Source: CAD feature listing. Evaluate the final solid. Frame: model axes, mm. A direction names the side the tool comes from. Round coordinates to 2 decimals unless told otherwise and drop trailing zeros. Loops run counter-clockwise (first coordinate to the right, second up) from the corner with the lowest first, then second, coordinate; pieces in that order, holes last.
Item 1: Section query C-C on y = -0.5. Return loops of the section in (x, z).
Item 2: Section query A-A on x = -23. Return loops of the section in (y, z), then the cut area to 3 significant figures.
Item 3: Section query D-D on z = 11. Give the number of separate pieces and of enclosed holes in the cut face, then the cut area to 3 significant figures.
Item 4: Pull-direction query (X, two-part tool) for faces 5 (the flat face through (14, 20, 13)), 6 (the cylindrical face through (7.18, 4.75, 11.9)), 7 (the flat face through (-26.86, 10.315, 48.479)); classes: released by +X, released by -X, zero draft, split by the parting line, or undercut.
Item 5: Access query for faces 1 (the flat face through (36, 28, 13)), 2 (the flat face through (31, -2.471, 48)), 3 (the flat face through (15, 18, 10)), 4 (the flat face through (36.1, 24.6, 50)). Directions: +Z, -Z, +X, -X, +Y, -Y. A direction counts if a zero-diameter tool reaches every point of the face in a straight line with its end or side. Return the directions, or none.
Item 6: Section query B-B on z = 39. Return loops of the section in (x, y).
Item 7: First-contact query: P1, Ø5, axis at x = 31, z = 10, coming from the +Y side; P2, Ø1.9, axis at x = 4.32, z = 11, coming from the -Y side; P3, Ø8, axis at x = 16.5, y = 21.5, coming from the -Z side; P4, Ø1, axis at x = 20.5, z = 14, coming from the +Y side. Flat tips, straight axial feed; report the tip coordinate or a pass-through.
Item 8: Ray query, L1, parallel to Z at x = 34, y = 26.5; L2, parallel to X at y = 1.5, z = 47.5 (3 decimals); L3, parallel to Z at x = 5, y = 11. Return the intervals inside material, ascending.
```python
from build123d import *

# Parameters (mm, degrees)
EXTRUDE_1_DEPTH     = 60
SKETCH_2_W          = 32.5
SKETCH_2_H          = 3
EXTRUDE_2_DEPTH     = 8.5
SKETCH_3_W          = 32.5
SKETCH_3_H          = 34
EXTRUDE_3_DEPTH     = 1
SKETCH_4_R          = 2.4
CUT_EXTRUDE_1_DEPTH = 100
CUT_EXTRUDE_3_DEPTH = 100
SKETCH_5_R          = 1.62
CUT_EXTRUDE_4_DEPTH = 100
SKETCH_7_R          = 3
CUT_EXTRUDE_5_DEPTH = 100


with BuildPart() as part:
    # 草图1 → 凸台-拉伸1 (new body)
    with BuildSketch(Plane.XY):
        Polygon((-38.683076923, -5.470769231), (45.316923077, -5.470769231), (45.244014743, 20.991341126), (44.341897344, 23.852491978), (-39.585194322, -2.609618379), align=None)
    extrude(amount=EXTRUDE_1_DEPTH)

    # 草图2 → 凸台-拉伸2 (add)
    with BuildSketch(Plane(origin=(-2.83104293, 8.978921042, 0), x_dir=(0.9537169507482267, 0.30070579950427384, 0), z_dir=(-0.30070579950427384, 0.9537169507482267, 0))):
        with Locations((-22.287798204, -11.5)):
            Rectangle(SKETCH_2_W, SKETCH_2_H)
        with Locations((-22.287798204, -48.5)):
            Rectangle(SKETCH_2_W, SKETCH_2_H)
        with Locations((33.212201796, -11.5)):
            Rectangle(SKETCH_2_W, SKETCH_2_H)
        with Locations((33.212201796, -48.5)):
            Rectangle(SKETCH_2_W, SKETCH_2_H)
    extrude(amount=EXTRUDE_2_DEPTH)

    # 草图3 → 凸台-拉伸3 (add)
    with BuildSketch(Plane(origin=(-2.83104293, 8.978921042, 0), x_dir=(0.9537169507482267, 0.30070579950427384, 0), z_dir=(-0.30070579950427384, 0.9537169507482267, 0))):
        with Locations((-22.287798204, -30)):
            Rectangle(SKETCH_3_W, SKETCH_3_H)
        with Locations((33.212201796, -30)):
            Rectangle(SKETCH_3_W, SKETCH_3_H)
    extrude(amount=EXTRUDE_3_DEPTH)

    # 草图4 → 切除-拉伸1 (cut)
    with BuildSketch(Plane.XY.offset(50)):
        with Locations((-35.850165862, 3.003309771)):
            Circle(SKETCH_4_R)
        with Locations((-14.874407062, 9.637911699)):
            Circle(SKETCH_4_R)
        with Locations((17.075110788, 19.711555982)):
            Circle(SKETCH_4_R)
        with Locations((38.056883705, 26.327083571)):
            Circle(SKETCH_4_R)
    extrude(amount=-CUT_EXTRUDE_1_DEPTH, mode=Mode.SUBTRACT)

    # 草图6 → 切除-拉伸3 (cut)
    with BuildSketch(Plane(origin=(0, 0, 10), x_dir=(-1, 0, 0), z_dir=(0, 0, -1))):
        Polygon((-31.771870066, 28.801675164), (-34.327869361, 20.695081083), (-23.360124428, 17.236964389), (-20.804125132, 25.34355847), align=None)
    extrude(amount=-CUT_EXTRUDE_3_DEPTH, mode=Mode.SUBTRACT)

    # 草图5 → 切除-拉伸4 (cut)
    with BuildSketch(Plane(origin=(0, -5.470769231, 0), x_dir=(-1, 0, 0), z_dir=(0, -1, 0))):
        with Locations(Location((-29.316923077, -49, 0), (0, 0, 180))):
            Circle(SKETCH_5_R)
        with Locations(Location((-29.316923077, -11, 0), (0, 0, 180))):
            Circle(SKETCH_5_R)
        with Locations(Location((-4.316923077, -49, 0), (0, 0, 180))):
            Circle(SKETCH_5_R)
        with Locations(Location((-4.316923077, -11, 0), (0, 0, 180))):
            Circle(SKETCH_5_R)
    extrude(amount=-CUT_EXTRUDE_4_DEPTH, mode=Mode.SUBTRACT)

    # 草图7 → 切除-拉伸5 (cut)
    with BuildSketch(Plane(origin=(0, -2.470769231, 0), x_dir=(-1, 0, 0), z_dir=(0, -1, 0))):
        with Locations(Location((-29.316923077, -11, 0), (0, 0, 180))):
            Circle(SKETCH_7_R)
        with Locations(Location((-4.316923077, -11, 0), (0, 0, 180))):
            Circle(SKETCH_7_R)
        with Locations(Location((-29.316923077, -49, 0), (0, 0, 180))):
            Circle(SKETCH_7_R)
        with Locations(Location((-4.316923077, -49, 0), (0, 0, 180))):
            Circle(SKETCH_7_R)
    extrude(amount=-CUT_EXTRUDE_5_DEPTH, mode=Mode.SUBTRACT)


solid = part.part
```
Data:
1. outline: (-40.25, 10) - (-32.89, 10) - (-32.89, 0) - (45.3, 0) - (45.3, 60) - (-32.89, 60) - (-32.89, 50) - (-40.25, 50) - (-40.25, 47) - (-36.22, 47) - (-36.22, 13) - (-40.25, 13) - close; hole circle Ø6 at (4.32, 11); hole circle Ø6 at (4.32, 49); hole circle Ø6 at (29.32, 11); hole circle Ø6 at (29.32, 49)
2. outline: (-5.47, 0) - (2.62, 0) - (2.62, 10) - (11.53, 10) - (11.53, 13) - (3.67, 13) - (3.67, 47) - (11.53, 47) - (11.53, 50) - (2.62, 50) - (2.62, 60) - (-5.47, 60) - close
2. area: 575 mm2
3. separate pieces: 3
3. enclosed holes: 4
3. area: 1,530 mm2
4. face 5: zero draft
4. face 6: undercut
4. face 7: released by -X
5. face 1: -X, +Y
5. face 2: +Y
5. face 3: -Z, -X, +Y
5. face 4: +Z, -X, +Y
6. outline: (-39.89, -1.66) - (-38.68, -5.47) - (45.32, -5.47) - (45.24, 20.99) - (44.04, 24.81) - (34.03, 21.65) - (34.33, 20.7) - (23.36, 17.24) - (23.06, 18.19) - (13.05, 15.03) - (13.35, 14.08) - (-8.59, 7.16) - (-8.89, 8.12) - close
7. P1: stops at y = 29.35
7. P2: passes through
7. P3: stops at z = 10
7. P4: stops at y = 17.54
8. L1: z = 10 to 13, 47 to 50
8. L2: x = -40.881 to -37.721, -33.979 to 1.719, 6.915 to 26.719, 31.915 to 45.298
8. L3: z = 0 to 8.08, 13.92 to 46.08, 51.92 to 60
